Part print with two shaded views. Sizes in mm from the minimum x, y, z corner. A direction names the side the tool comes from. Coordinates: 2 decimals unless noted, no trailing zeros. Write each loop counter-clockwise with the first axis right and the second up, starting at its lowest first coordinate (ties: lowest second). Pieces come first, ordered by that corner, then holes. Notation, with made-up numbers: (17.25, 37.5) -> (32.25, 37.5) arc R9 ccw to (32.25, 44.5) -> close; hole circle Ø5 at (87, -19). An arc over 180 degrees is marked (long way). Write item = value, one per line. Start each with the question number.
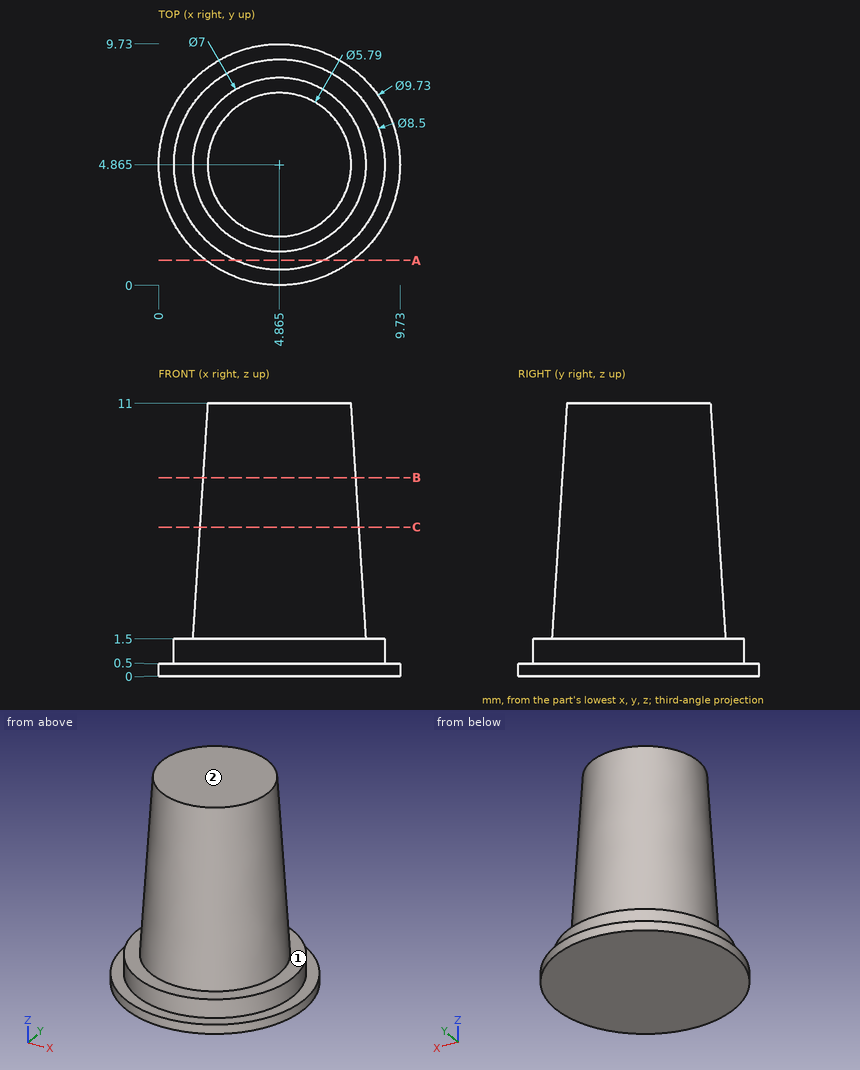
(1) Drill centre lines: line 1 along Z through (x, y) = (4, 8.75); line 2 along Z through (x, y) = (1.75, 1.75); line 3 along X through (y, z) = (4.75, 0.75). Where is each one in solid material? Low to high.
(2) Saw through at C-C (z = 6). Give the cut face in (x, y) (3 decimals), then the cut area to 3 significant figures.
(3) Saw through at A-A (y = 1). Give the cut face in (x, z), then the cut area to 3 significant figures.
(4) Drop flat-ended pins along their axis: pin 1 Ø3 at (y, z) = (5.5, 7) entering from +X; pin 2 Ø1.5 at (x, z) = (4.5, 8) entering from -Y; pin 3 Ø5 at (x, z) = (8, 2.5) entering from -Y. Give the stop position or say it passes through.
(5) Saw through at B-B (z = 8). Give the cut face in (x, y) (3 decimals).
(6) 3-axis set-ups, long thin cutter, end or side, ignore diameter. For the marked faces 1 and 2: which of +Z, -Z, +X, -X, +Y, -Y reach the whole face in a straight line?
Returned:
q1.line_1 = 0 to 1.5
q1.line_2 = 0 to 0.5
q1.line_3 = 0.62 to 9.11
q2.outline = circle Ø6.427 at (4.865, 4.865)
q2.area = 32.4 mm2
q3.outline = (1.91, 0) -> (7.82, 0) -> (7.82, 0.5) -> (6.63, 0.5) -> (6.63, 1.5) -> (3.1, 1.5) -> (3.1, 0.5) -> (1.91, 0.5) -> close
q3.area = 6.49 mm2
q4.pin_1 = 8.1
q4.pin_2 = 1.74
q4.pin_3 = 0.28
q5.outline = circle Ø6.172 at (4.865, 4.865)
q6.face_1 = +Z
q6.face_2 = +Z, +X, -X, +Y, -Y
